Work out the finished part from the listing and answer in its coordinate system (mm). A direction names the side the tool comes from. Coordinates: 2 decimals unless noted, no trailing zeros. Write each loop counter-clockwise with the first axis right and the second up, starting at its lowest first coordinate (ties: lowest second). Pieces come first, ordered by that corner, then holes. Notation, with made-up numbers: M 10,-2.5 L 27,-2.5 A24 cw 27,12.5 Z; hole C -31.75,39 d9. An arc over 180 degrees is marked long. Answer as CSV lines item,"result". Start each with the question number.
(1) For faces 1 (the flat face through (42.93, -0.07, 36.12)), 2 (the flat face through (-1, 22, 5)), 3 (the flat face through (-1, -5, 33)), determine the directions among +Z, -Z, +X, -X, +Y, -Y from which every point of the face is accessible in a straight line to the end or side of a thin tool.
(2) Flat-ended cylindrical pins translate along their axes: P1, Ø4, axis at x = 17.5, z = 31, coming from the -Y side; P2, Ø12, axis at x = -5.5, y = 27, coming from the +Z side; P3, Ø5, axis at x = -28.5, y = 2, coming from the +Z side. Find the tip coordinate at first contact, or state that the pin passes through.
(3) A cutting plane is placed at D-D on x = -34.5. Give the vertices of the cut face in (y, z), then the cut area to 3 significant figures.
(4) A cutting plane is placed at A-A on x = 52.5. Give the vertices of the cut face in (y, z), then the cut area to 3 significant figures.
(5) Find the intervals of material crossed by L1, parallel to Y at x = -50, z = 1.55; L2, parallel to Y at x = 44, z = 24, in increasing order. Write a range as [from, to].
(6) A cutting plane is placed at C-C on z = 47. Give the vertices of the cut face in (x, y), then the cut area to 3 significant figures.
(7) The mould has two halves that part along Z. Classify faces 4 (the flat face through (-70, 0, 0)), 5 (the flat face through (-1, -23, 5)), 6 (the cylindrical face through (-1.627, 0.07, 67.394)): released by +Z, released by -Z, zero draft, split by the parting line, or undercut.
(8) A cutting plane is placed at B-B on y = -28. Give the vertices of the cut face in (x, z), then the cut area to 3 significant figures.
from build123d import *

# Parameters (mm, degrees)
F0_W     = 140
F0_H     = 10
F1_DEPTH = 40
F0_R     = 12.5
F2_DEPTH = 5
F3_R     = 20
F5_D     = 20
F5_DEPTH = 5.001
F6_D     = 20
F7_D     = 20
F7_DEPTH = 5.001
F8_D     = 20
F9_D     = 20
F9_DEPTH = 5.001
F10_D    = 20


with BuildPart() as f1:
    # F0 (on Front) → F1 (new body, symmetric)
    with BuildSketch(Plane.XZ):
        Rectangle(F0_W, F0_H)
    extrude(amount=F1_DEPTH, both=True)

    # F0 (on Front) → F2 (join, symmetric)
    with BuildSketch(Plane.XZ):
        Rectangle(F0_W, F0_H)
        with BuildLine():
            Line((-70, 5), (70, 5))
            Line((70, 5), (15.0900003586, 68.126000502))
            ThreePointArc((15.0900003586, 68.126000502), (0, 75), (-15.0900003586, 68.126000502))
            Line((-15.0900003586, 68.126000502), (-70, 5))
        make_face()
        with Locations((0, 55)):
            Circle(F0_R, mode=Mode.SUBTRACT)
    extrude(amount=F2_DEPTH, both=True)

    # F3
    f3_edges = [f1.edges().sort_by_distance(p)[0] for p in [
        (-70, 40, 0),
        (-70, -40, 0),
        (70, 40, 0),
        (70, -40, 0),
    ]]
    fillet(f3_edges, radius=F3_R)

    # F5 (through all, one way)
    with BuildSketch(Plane.XY):
        with Locations((52.5, 22.5)):
            Circle(F5_D / 2)
    extrude(amount=-F5_DEPTH, mode=Mode.SUBTRACT)

    # F6 (through all)
    with Locations(Plane(origin=(0, 0, 0), x_dir=(1, 0, 0), z_dir=(0, 0, -1))):
        with Locations((52.5, -22.5)):
            Hole(F6_D / 2)

    # F7 (through all, one way)
    with BuildSketch(Plane.XY):
        with Locations((-50, 20)):
            Circle(F7_D / 2)
    extrude(amount=-F7_DEPTH, mode=Mode.SUBTRACT)

    # F8 (through all)
    with Locations(Plane(origin=(0, 0, 0), x_dir=(1, 0, 0), z_dir=(0, 0, -1))):
        with Locations((-50, -20)):
            Hole(F8_D / 2)

    # F9 (through all, one way)
    with BuildSketch(Plane.XY):
        with Locations((-50, -20), (52.5, -20)):
            Circle(F9_D / 2)
    extrude(amount=-F9_DEPTH, mode=Mode.SUBTRACT)

    # F10 (through all)
    with Locations(Plane(origin=(0, 0, 0), x_dir=(1, 0, 0), z_dir=(0, 0, -1))):
        with Locations((-50, 20), (52.5, 20)):
            Hole(F10_D / 2)


solid = f1.part
Here are the results:
1,face 1,"+Z, +X, +Y, -Y"
1,face 2,"+Z, +X, -X, +Y"
1,face 3,"+Z, +X, -X, -Y"
2,P1,"stops at y = -5"
2,P2,"stops at z = 5"
2,P3,"stops at z = 55.58"
3,outline,"M -40,-5 L 40,-5 L 40,5 L 5,5 L 5,45.81 L -5,45.81 L -5,5 L -40,5 Z"
3,area,"1,210 mm^2"
4,outline,"M -39.84,-5 L -30,-5 L -30,5 L -39.84,5 Z; M -10,-5 L 12.5,-5 L 12.5,5 L 5,5 L 5,25.12 L -5,25.12 L -5,5 L -10,5 Z; M 32.5,-5 L 39.84,-5 L 39.84,5 L 32.5,5 Z"
4,area,"598 mm^2"
5,L1,"y = [-40, -30], [-10, 10], [30, 40]"
5,L2,"y = [-5, 5]"
6,outline,"M -33.47,-5 L -9.6,-5 L -9.6,5 L -33.47,5 Z; M 9.6,-5 L 33.47,-5 L 33.47,5 L 9.6,5 Z"
6,area,"477 mm^2"
7,face 4,"zero draft"
7,face 5,"released by +Z"
7,face 6,"undercut"
8,outline,"M -68.33,-5 L -56,-5 L -56,5 L -68.33,5 Z; M -44,-5 L 46.5,-5 L 46.5,5 L -44,5 Z; M 58.5,-5 L 68.33,-5 L 68.33,5 L 58.5,5 Z"
8,area,"1,130 mm^2"
